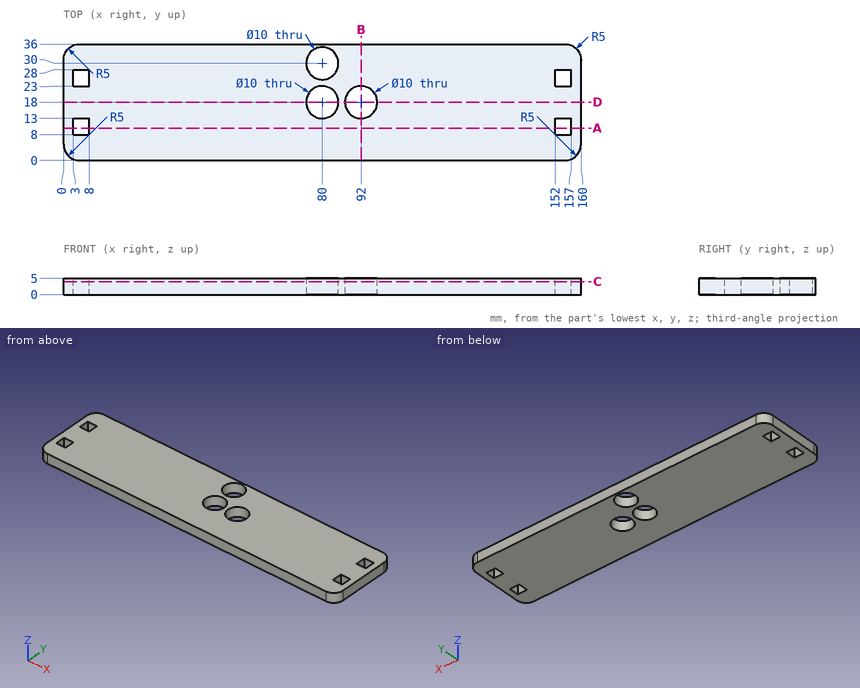
Study the drawing (mm; zero at the part's minimum x, y, z) and answer. Coordinates: 2 decimals unless noted, no trailing zeros. Write each loop counter-clockwise with the first axis right and the second up, starting at its lowest first coordinate (ties: lowest second). Pieces come first, ordered by that corner, then holes. Notation, with made-up numbers: (33, -28) - (41, -28) arc R16 cw to (41, -24) - close; hole circle Ø3 at (76.25, -3.5). An arc over 180 degrees is marked (long way). One line per item, written item: value.
1) Consider line 1 along Y through (x, z) = (80, 3.2); line 2 along X through (y, z) = (12, 4.7); line 3 along Y through (x, z) = (78.5, 1.6). Determine where each line is inside the solid, lowest interval first. Write a range as from..to.
Geometry check:
line 1: y = 0..13, 23..25, 35..36
line 2: x = 0..3, 8..152, 157..160
line 3: y = 0..13.23, 22.77..25.23, 34.77..36
2) Find section A-A (y = 10). Give the vertices of the cut face in (x, z).
Geometry check:
outline: (0, 0) - (3, 0) - (3, 5) - (0, 5) - close; (8, 0) - (152, 0) - (152, 5) - (8, 5) - close; (157, 0) - (160, 0) - (160, 5) - (157, 5) - close
3) Find section D-D (y = 18). Give the vertices of the cut face in (x, z), and give its area (3 significant figures).
Geometry check:
outline: (0, 0) - (75, 0) - (75, 5) - (0, 5) - close; (85, 0) - (87, 0) - (87, 5) - (85, 5) - close; (97, 0) - (160, 0) - (160, 5) - (97, 5) - close
area: 700 mm2
4) Find section C-C (z = 4). Give the vertices of the cut face in (x, y), and give its area (3 significant figures).
Geometry check:
outline: (0, 5) arc R5 ccw to (5, 0) - (155, 0) arc R5 ccw to (160, 5) - (160, 31) arc R5 ccw to (155, 36) - (5, 36) arc R5 ccw to (0, 31) - close; hole (3, 8) - (8, 8) - (8, 13) - (3, 13) - close; hole (3, 23) - (8, 23) - (8, 28) - (3, 28) - close; hole circle Ø10 at (80, 18); hole circle Ø10 at (80, 30); hole circle Ø10 at (92, 18); hole (152, 8) - (157, 8) - (157, 13) - (152, 13) - close; hole (152, 23) - (157, 23) - (157, 28) - (152, 28) - close
area: 5,400 mm2
5) This flat-tipped pin is pushed along its axis until it touches: pin 1 Ø8 at (x, y) = (80, 30) entering from -Z. Where does it stop, or does it pass through?
Geometry check:
pin 1: passes through
6) Find section B-B (x = 92). Give the vertices of the cut face in (y, z), and give its area (3 significant figures).
Geometry check:
outline: (0, 0) - (13, 0) - (13, 5) - (0, 5) - close; (23, 0) - (36, 0) - (36, 5) - (23, 5) - close
area: 130 mm2
